Autodesk Inventor part; units mm, degrees
ref_plane "YZ Plane" through (0, 0, 0) normal (1, 0, 0) x (0, 1, 0)
ref_plane "XZ Plane" through (0, 0, 0) normal (0, 1, 0) x (-1, 0, 0)
ref_plane "XY Plane" through (0, 0, 0) normal (0, 0, 1) x (1, 0, 0)
sketch "Sketch1" plane through (0, 0, 0) normal (0, 1, 0) x (-1, 0, 0)
  line L0 (105, -150) -> (-105, -150)
  line L1 (-105, -150) -> (-105, 150)
  line L2 (-105, 150) -> (105, 150)
  line L3 (105, 150) -> (105, -150)
  line L4 (105, -150) -> (-105, 150) construction
  line L5 (-105, -150) -> (105, 150) construction
  point P0 (0, 0)
  dimension "d0" = 210
  dimension "d1" = 300
extrude "Extrusion1" add sketch "Sketch1" along normal blind 30
sketch "Sketch2" plane through (0, 30, 0) normal (0, 1, 0) x (1, 0, 0)
  circle A0 centre (0, 100) radius 9
  circle A1 centre (0, -100) radius 9
  point P0 (0, 0)
  dimension "d4" = 18
  dimension "d5" = 18
  dimension "d6" = 100
  dimension "d7" = 100
hole "Hole1" at (0, 30, -100) at (0, 30, 100) direction (0, -1, 0) diameter 0.1 end through all counterbore diameter 18 counterbore depth 24
sketch "Sketch3" plane through (0, 30, 0) normal (0, 1, 0) x (1, 0, 0)
  line L0 (65, -145) -> (100, -145)
  line L1 (100, -145) -> (100, -85)
  line L2 (100, -85) -> (65, -85)
  line L3 (65, -85) -> (65, -145)
  line L4 (-105, -150) -> (105, -150)
  line L5 (105, -150) -> (105, 150)
  point P0 (0, 0)
  dimension "d15" = 35
  dimension "d16" = 60
  dimension "d17" = 5
  dimension "d19" = 5
extrude "Extrusion2" cut sketch "Sketch3" against normal blind 3.5
fillet "Fillet1" radius 4 4 edges at (105, 15, 150) (-105, 15, 150) (105, 15, -150) (-105, 15, -150)
properties part number "Podstawa"
Can you work these out from the model? Positions are in its coordinate system, mm. A direction names the side the tool comes from. Round coordinates to 2 decimals unless told otherwise and drop trailing zeros. Loops run counter-clockwise (first coordinate to the right, second up) from the corner with the lowest first, then second, coordinate; pieces in that order, holes last. Notation, with made-up numbers: M 0,48 L 9,48 A18 ccw 9,57 Z; hole C 45.5,9.25 d7. An arc over 180 degrees is marked long. Write item = value, one per line. Start each with the question number.
(1) If we mould it in two halves opening along Z, with no side actions, what happens to faces 3 (the face through (-1, 15, -150)), 4 (the face through (2, 6, 100)), 5 (the face through (-105, 15, 2))? For each: released by +Z, released by -Z, zero draft, split by the parting line, or undercut.
(2) I need wall thicknesses on line 1 along Z through (x, y) = (0, 21.5); line 2 along Y through (x, z) = (82, 109.5). Which ranges of each line are inside material? Lowest first, please.
(3) Which directions (+Z, -Z, +X, -X, +Y, -Y) give clear straight access to the entire face, cutting with the end or side of a thin tool? Please do faces 1 (the face through (1, 0, 2)), 2 (the face through (-2.703, 17.832, -91.416)).
(4) I'm going to push a flat-ended pin straight in: P1, Ø10.5, axis at x = 75.5, z = 106, coming from the +Y side. Where does the tip first touch, or does it pass through?
(5) Suppose I cut it at A-A on x = 88.5. Write out the boundary of the cut face in (y, z).
Answer block:
q1.face_3 = released by -Z
q1.face_4 = undercut
q1.face_5 = zero draft
q2.line_1 = -150 to -109, -91 to 91, 109 to 150
q2.line_2 = 0 to 26.5
q3.face_1 = +Z, -Z, +X, -X, -Y
q3.face_2 = +Y
q4.P1 = 26.5
q5.outline = M 0,-150 L 30,-150 L 30,85 L 26.5,85 L 26.5,145 L 30,145 L 30,150 L 0,150 Z
